Autodesk Inventor part; units mm, degrees
ref_plane "YZ Plane" through (0, 0, 0) normal (1, 0, 0) x (0, 1, 0)
ref_plane "XZ Plane" through (0, 0, 0) normal (0, 1, 0) x (-1, 0, 0)
ref_plane "XY Plane" through (0, 0, 0) normal (0, 0, 1) x (1, 0, 0)
ref_plane "Work Plane1" through (0, 0, 0) normal (0, 0, 1) x (1, 0, 0)
sketch "Sketch1" plane through (0, 0, 0) normal (0, 0, 1) x (1, 0, 0)
  line L0 (3.99, 16.87) -> (-0.09, 16.87)
  line L1 (-3.99, 20.77) -> (-0.09, 16.87)
  line L2 (-3.99, 24.85) -> (-3.99, 20.77)
  line L3 (-37.73, 24.85) -> (-3.99, 24.85)
  line L4 (-37.73, 16.87) -> (-37.73, 24.85)
  line L5 (-45.71, 16.87) -> (-37.73, 16.87)
  line L6 (-45.71, -16.87) -> (-45.71, -13.8689)
  line L7 (-41.63, -16.87) -> (-45.71, -16.87)
  line L8 (-37.73, -20.77) -> (-41.63, -16.87)
  line L9 (-37.73, -20.77) -> (-37.73, -24.85)
  line L10 (-37.73, -24.85) -> (-3.99, -24.85)
  line L11 (-3.99, -24.85) -> (-3.99, -20.77)
  line L12 (-0.09, -16.87) -> (-3.99, -20.77)
  line L13 (-0.09, -16.87) -> (3.99, -16.87)
  line L14 (3.99, -16.87) -> (3.99, 16.87)
  arc A0 (-35.53, 10.1) -> (-37.83, 7.8) centre (-35.53, 7.8) ccw
  line L15 (-37.83, -16.97) -> (-37.83, 16.97) construction
  arc A1 (-37.83, -7.8) -> (-35.53, -10.1) centre (-35.53, -7.8) ccw
  arc A2 (-19.93, -10.1) -> (-17.63, -7.8) centre (-19.93, -7.8) ccw
  arc A3 (-17.63, 7.8) -> (-19.93, 10.1) centre (-19.93, 7.8) ccw
  line L16 (-37.83, -7.8) -> (-37.83, 7.8)
  line L17 (-35.53, 10.1) -> (-19.93, 10.1)
  line L18 (-17.63, 7.8) -> (-17.63, -7.8)
  line L19 (-35.53, -10.1) -> (-19.93, -10.1)
  circle A4 centre (-27.73, 0) radius 8.4
  line L20 (-45.71, 13.8689) -> (-40.3869, 13.8689)
  line L21 (-40.3869, 13.8689) -> (-34.7289, 19.5269)
  line L22 (-34.7289, 19.5269) -> (-8.86, 19.5269)
  line L23 (-8.86, 19.5269) -> (-8.86, -19.5269)
  line L24 (-8.86, -19.5269) -> (-34.7289, -19.5269)
  line L25 (-34.7289, -19.5269) -> (-40.3869, -13.8689)
  line L26 (-40.3869, -13.8689) -> (-45.71, -13.8689)
  line L27 (-45.71, 13.8689) -> (-45.71, 16.87)
  point P0 (0, 0)
  point P1 (-17.63, -7.8)
extrude "Extrusion1" add sketch "Sketch1" along normal blind 9 contours L17 A3 L18 A2 L19 A1 L16 A0
sketch "Sketch2" plane through (0, 0, 9) normal (0, 0, 1) x (1, 0, 0)
  circle A0 centre (-20.86, 0) radius 16.97 construction
  line L0 (-19.93, 10.1) -> (-35.53, 10.1)
  arc A1 (-35.53, 10.1) -> (-37.83, 7.8) centre (-35.53, 7.8) ccw
  line L1 (-37.83, 7.8) -> (-37.83, -7.8)
  arc A2 (-37.83, -7.8) -> (-35.53, -10.1) centre (-35.53, -7.8) ccw
  line L2 (-35.53, -10.1) -> (-19.93, -10.1)
  arc A3 (-19.93, -10.1) -> (-17.63, -7.8) centre (-19.93, -7.8) ccw
  line L3 (-17.63, -7.8) -> (-17.63, 7.8)
  arc A4 (-17.63, 7.8) -> (-19.93, 10.1) centre (-19.93, 7.8) ccw
  point P0 (0, 0)
hole "Hole1" at (-35.53, -7.8, 9) at (-35.53, 7.8, 9) direction (0, 0, -1) diameter 2.2 depth 15 tip angle 118
sketch "Sketch3" plane through (0, 0, 0) normal (0, 0, -1) x (-1, 0, 0)
  circle A0 centre (27.73, 0) radius 8.4
  circle A1 centre (27.73, 0) radius 9.25
  circle A2 centre (27.73, 0) radius 9.15
  point P0 (0, 0)
  dimension "d10" = 0.1
extrude "Extrusion2" add sketch "Sketch3" along normal blind 2 contours A2
properties part number "30_Cube_SQUID_Z_Focus_spacer_v3"
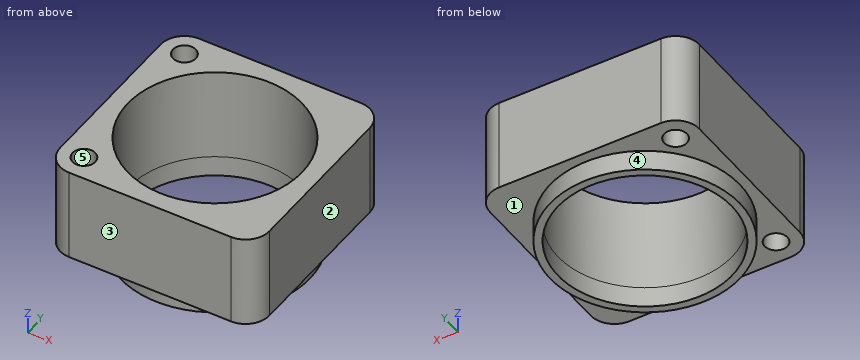
Design review of the part built by this model. Coordinates are the model's own, in mm. Face numbers are marked on the shaded views. A direction names the side the tool comes from. Round coordinates to 2 decimals unless told otherwise and drop trailing zeros. Loops run counter-clockwise (first coordinate to the right, second up) from the corner with the lowest first, then second, coordinate; pieces in that order, holes last. Notation, with made-up numbers: (-32, 81.5) - (-24, 81.5) arc R29 ccw to (-24, 102.5) - close; hole circle Ø4 at (-29, -23). An arc over 180 degrees is marked (long way). One line per item, written item: value. Start each with the question number.
1) For the marked faces 1 and 2, list the 3-axis set-ups (+Z, -Z, +X, -X, +Y, -Y) from which the entire face can be reached by the end or side of a thin tool; tool diameter is ignored.
2) Consider section D-D on z = -0.75. Give the boundary of the cut face in (x, y).
3) Consider section C-C on z = 0.75. Give the boundary of the cut face in (x, y), then the cut area to 3 significant figures.
4) Consider section B-B on x = -27.73. Give the boundary of the cut face in (y, z), then the cut area to 3 significant figures.
5) Draft analysis for pull direction X (two halves, no side actions). For the marked faces 3, 4 and 5, state which applies: +X half, -X half, draft (parallel to the pull), parting line (faces both ways), or undercut.
6) Insertion check: pin 1 Ø6 at (x, y) = (-26, -5.5) entering from -Z; pin 2 Ø1.8 at (x, y) = (-35.53, -7.8) entering from -Z. Each pin has a flat end and moves straight along its axis. Give the tip position at first contact, or say it passes through.
7) Consider section A-A on y = 0. Give the boundary of the cut face in (x, z), then the cut area to 3 significant figures.
8) To check wall thickness, follow L1, parallel to Y at x = -27.73, z = 6; L2, parallel to X at y = 0, z = 6.25; L3, parallel to Y at x = -36.25, z = 7.25. State the ranges of each line that lie inside material, in increasing order. Write a range as from..to.
Reported:
1. face 1: -Z
1. face 2: +Z, -Z, +X, +Y, -Y
2. outline: circle Ø18.3 at (-27.73, 0); hole circle Ø16.8 at (-27.73, 0)
3. outline: (-37.83, -7.8) arc R2.3 ccw to (-35.53, -10.1) - (-19.93, -10.1) arc R2.3 ccw to (-17.63, -7.8) - (-17.63, 7.8) arc R2.3 ccw to (-19.93, 10.1) - (-35.53, 10.1) arc R2.3 ccw to (-37.83, 7.8) - close; hole circle Ø2.2 at (-35.53, -7.8); hole circle Ø2.2 at (-35.53, 7.8); hole circle Ø16.8 at (-27.73, 0)
3. area: 174 mm^2
4. outline: (-10.1, 0) - (-9.15, 0) - (-9.15, -2) - (-8.4, -2) - (-8.4, 9) - (-10.1, 9) - close; (8.4, -2) - (9.15, -2) - (9.15, 0) - (10.1, 0) - (10.1, 9) - (8.4, 9) - close
4. area: 33.6 mm^2
5. face 3: draft
5. face 4: parting line
5. face 5: undercut
6. pin 1: stops at z = -2
6. pin 2: passes through
7. outline: (-37.83, 0) - (-36.88, 0) - (-36.88, -2) - (-36.13, -2) - (-36.13, 9) - (-37.83, 9) - close; (-19.33, -2) - (-18.58, -2) - (-18.58, 0) - (-17.63, 0) - (-17.63, 9) - (-19.33, 9) - close
7. area: 33.6 mm^2
8. L1: y = -10.1..-8.4, 8.4..10.1
8. L2: x = -37.83..-36.13, -19.33..-17.63
8. L3: y = -9.98..-8.63, -6.97..6.97, 8.63..9.98
